Read the model definition and answer for the solid it produces. Units are mm, in the model's axes. A direction names the side the tool comes from. Coordinates: 2 decimals unless noted, no trailing zeros. Loops run counter-clockwise (first coordinate to the right, second up) from the corner with the lowest first, then second, coordinate; pieces in that order, holes last. Notation, with made-up numbers: M 30.5,-37 L 70.5,-37 A20 cw 70.5,-11 Z; hole C -15,17.5 d5. An arc over 180 degrees is marked long. One line per item, written item: value. Start each with the question number.
1. Consider probe 1 along Z at (x, y) = (-19, 2.5); probe 2 along Z at (x, y) = (15, -23); probe 3 along X at (y, z) = (-4, 25). Determine where each line is inside the solid, lowest interval first.
2. Determine the mould class of faces 1 (the face through (-11.19, -21.514, 19.919)), 2 (the face through (2.124, -9.567, 30.231)), 3 (the face through (0, -1, 40)) for opening direction Z: +Z half, -Z half, draft (parallel to the pull), parting line (faces both ways), or undercut.
3. Flat-ended cylindrical pins translate along their axes: pin 1 (18 mm diameter, centred on x = 14.5, y = 8.5, fed in from -Z); pin 2 (2.5 mm diameter, centred on x = -1, z = 36, fed in from +Y); pin 3 (1.5 mm diameter, centred on y = -7, z = 13, fed in from -X). Find the tip coordinate at first contact, or state that the pin passes through.
4. The part is cut by section B-B (z = 30). Write down the section's boundary in (x, y).
5. For faces 4 (the face through (0, 2.9, 36)), 5 (the face through (0, 4, 31.6)), 6 (the face through (7.1, 7.1, 10.9)), 7 (the face through (0, 2.9, 4)), determine the directions among +Z, -Z, +X, -X, +Y, -Y from which every point of the face is accessible in a straight line to the end or side of a thin tool.
6. The part is cut by section A-A (x = 0). Write down the section's boundary in (y, z).
```python
from build123d import *

# Parameters (mm, degrees)
EXTRUDE_1_DEPTH      = 40
SKETCH_2_R           = 9.8
EXTRUDE_2_DEPTH      = 23.4
EXTRUDE_3_DEPTH      = 9
EXTRUDE_3_DEPTH_BACK = 9
SKETCH_3_R           = 30
EXTRUDE_4_DEPTH      = 2
EXTRUDE_4_DEPTH_BACK = 2
SKETCH_5_R           = 24.25


with BuildPart() as part:
    # 스케치1 → 보스-돌출1 (new body)
    with BuildSketch(Plane.XY):
        with BuildLine():
            Line((3.8249183, 2.9), (-3.8249183, 2.9))
            ThreePointArc((-3.8249183, 2.9), (-1.529769944, -4.549703718), (4.8, 0))
            ThreePointArc((4.8, 0), (4.549703718, 1.529769944), (3.8249183, 2.9))
        make_face()
    extrude(amount=EXTRUDE_1_DEPTH)

    # 스케치2 → 보스-돌출2 (add)
    with BuildSketch(Plane(origin=(0, 0, 8.2), x_dir=(-1, 0, 0), z_dir=(0, 0, -1))):
        Circle(SKETCH_2_R)
    extrude(amount=-EXTRUDE_2_DEPTH)

    # 스케치3 → 보스-돌출3 (add, two sides: drawn at the far end of the back side and taken through both)
    with BuildSketch(Plane(origin=(0, 0, 19.9), x_dir=(-1, 0, 0), z_dir=(0, 0, -1)).offset(-EXTRUDE_3_DEPTH_BACK)):
        Circle(SKETCH_3_R)
    extrude(amount=EXTRUDE_3_DEPTH + EXTRUDE_3_DEPTH_BACK)

    # 스케치4 → 컷-회전1 (revolve, cut)
    with BuildSketch(Plane(origin=(0, 0, 0), x_dir=(0, 0, -1), z_dir=(1, 0, 0)), mode=Mode.PRIVATE) as cut_revolve_1_sk:
        Polygon((-19.9, 23), (-12.4, 30), (-27.4, 30), align=None)
    revolve(cut_revolve_1_sk.sketch.rotate(Axis((0, 0, -4.267978706), (0, 0, 1)), 90), axis=Axis((0, 0, -4.267978706), (0, 0, 1)), mode=Mode.SUBTRACT)

    # 스케치5 → 보스-돌출4 (add, two sides: drawn at the far end of the back side and taken through both)
    with BuildSketch(Plane(origin=(0, 0, 19.9), x_dir=(-1, 0, 0), z_dir=(0, 0, -1)).offset(-EXTRUDE_4_DEPTH_BACK)):
        Circle(SKETCH_5_R)
    extrude(amount=EXTRUDE_4_DEPTH + EXTRUDE_4_DEPTH_BACK)


solid = part.part
```
Answer block:
1. probe 1: z = 10.9 to 28.9
1. probe 2: z = 10.9 to 15.12, 24.68 to 28.9
1. probe 3: x = -27.47 to 27.47
2. face 1: undercut
2. face 2: draft
2. face 3: +Z half
3. pin 1: stops at z = 8.2
3. pin 2: stops at y = 2.9
3. pin 3: stops at x = -29.28
4. outline: C 0,0 d19.6
5. face 4: +Z, +X, -X, +Y
5. face 5: +Z
5. face 6: -Z
5. face 7: -Z, +X, -X, +Y
6. outline: M -30,10.9 L -9.8,10.9 L -9.8,8.2 L -4.8,8.2 L -4.8,0 L 2.9,0 L 2.9,8.2 L 9.8,8.2 L 9.8,10.9 L 30,10.9 L 30,12.4 L 24.25,18.56 L 24.25,21.24 L 30,27.4 L 30,28.9 L 9.8,28.9 L 9.8,31.6 L 2.9,31.6 L 2.9,40 L -4.8,40 L -4.8,31.6 L -9.8,31.6 L -9.8,28.9 L -30,28.9 L -30,27.4 L -24.25,21.24 L -24.25,18.56 L -30,12.4 Z
